Could you check a few things on this model? Use its own coordinates, in mm. A direction names the side the tool comes from. Give positions to 0.01 mm unless a question says otherwise; leave off trailing zeros. Loops run counter-clockwise (first coordinate to the right, second up) from the corner with the lowest first, then second, coordinate; pieces in that order, holes last. Notation, with made-up numbers: (-30, 3.5) - (25, 3.5) arc R14 ccw to (25, 23.5) - close; hole circle Ø2 at (27.5, -26.5). An arc over 180 degrees is marked (long way). One line per item, written item: value. Start each with the question number.
Q1. I want a section at B-B (x = 4). Please give me the cut outline in (y, z), then the cut area to 3 significant figures.
Q2. For faces 1 (the face through (11, 1, 2)), 2 (the face through (0, -38, 2)), which set-ups out of +Z, -Z, +X, -X, +Y, -Y let a thin tool reach every point of the face, with its end or its side?
Q3. I want a section at A-A (y = -40.5). Please give me the cut outline in (x, z).
Q4. If I drill on line 1 (Y direction, x = -8, z = 0.3); line 2 (Y direction, x = 5.5, z = 1.55); line 3 (X direction, y = 33.5, z = 2.25), over which ranges is the centre line in solid material (lowest first)? Write a range as from..to.
Q5. I want a section at C-C (y = 29.5). Please give me the cut outline in (x, z), then the cut area to 3 significant figures.
Q6. I want a section at D-D (z = 0.8). Please give me the cut outline in (x, y).
Autodesk Inventor part; units mm, degrees
ref_plane "YZ Plane" through (0, 0, 0) normal (1, 0, 0) x (0, 1, 0)
ref_plane "XZ Plane" through (0, 0, 0) normal (0, 1, 0) x (-1, 0, 0)
ref_plane "XY Plane" through (0, 0, 0) normal (0, 0, 1) x (1, 0, 0)
sketch "Sketch1" plane through (0, 0, 0) normal (0, 0, 1) x (1, 0, 0)
  line L0 (-11, 43) -> (11, 43)
  line L1 (11, 43) -> (11, -43)
  line L2 (11, -43) -> (-11, -43)
  line L3 (-11, -43) -> (-11, 43)
  line L4 (-11, 43) -> (11, -43) construction
  line L5 (11, 43) -> (-11, -43) construction
  circle A0 centre (-8, 40.5) radius 1.5
  circle A1 centre (8, 40.5) radius 1.5
  circle A2 centre (-8, -40.5) radius 1.5
  circle A3 centre (8, -40.5) radius 1.5
  line L6 (7, 38) -> (-7, 38)
  line L7 (-7, 38) -> (-7, -38)
  line L8 (-7, -38) -> (7, -38)
  line L9 (7, -38) -> (7, 38)
  line L10 (7, 38) -> (-7, -38) construction
  line L11 (-7, 38) -> (7, -38) construction
  point P0 (0, 0)
  dimension "d0" = 22
  dimension "d1" = 86
  dimension "d2" = 3
  dimension "d3" = 3
  dimension "d4" = 3
  dimension "d5" = 3
  dimension "d6" = 3
  dimension "d7" = 2.5
  dimension "d8" = 3
  dimension "d9" = 2.5
  dimension "d10" = 2.5
  dimension "d11" = 3
  dimension "d12" = 3
  dimension "d13" = 2.5
  dimension "d14" = 14
  dimension "d15" = 76
extrude "Extrusion1" add sketch "Sketch1" along normal blind 4
properties part number "PartC" material "Aluminum 6061"
Worked answers:
1. outline: (-43, 0) - (-38, 0) - (-38, 4) - (-43, 4) - close; (38, 0) - (43, 0) - (43, 4) - (38, 4) - close
1. area: 40.0 mm²
2. face 1: +Z, -Z, +X, +Y, -Y
2. face 2: +Z, -Z
3. outline: (-11, 0) - (-9.5, 0) - (-9.5, 4) - (-11, 4) - close; (-6.5, 0) - (6.5, 0) - (6.5, 4) - (-6.5, 4) - close; (9.5, 0) - (11, 0) - (11, 4) - (9.5, 4) - close
4. line 1: y = -43..-42, -39..39, 42..43
4. line 2: y = -43..-38, 38..43
4. line 3: x = -11..-7, 7..11
5. outline: (-11, 0) - (-7, 0) - (-7, 4) - (-11, 4) - close; (7, 0) - (11, 0) - (11, 4) - (7, 4) - close
5. area: 32.0 mm²
6. outline: (-11, -43) - (11, -43) - (11, 43) - (-11, 43) - close; hole circle Ø3 at (-8, -40.5); hole circle Ø3 at (-8, 40.5); hole (-7, -38) - (7, -38) - (7, 38) - (-7, 38) - close; hole circle Ø3 at (8, -40.5); hole circle Ø3 at (8, 40.5)
